Can you work these out from the model? Positions are in its coordinate system, mm. Face numbers are marked on the shaded views. Give positions to 0.01 mm unless a question says otherwise; leave off trailing zeros. Loops run counter-clockwise (first coordinate to the right, second up) from the corner with the lowest first, then second, coordinate; pieces in that order, holes last. Notation, with made-up numbers: (-7.5, 13.5) - (17.5, 13.5) arc R33 ccw to (17.5, 48.5) - close; hole circle Ø3 at (46, 32.25). An arc over 180 degrees is marked (long way). Answer as a JSON object with one key per item and string values.
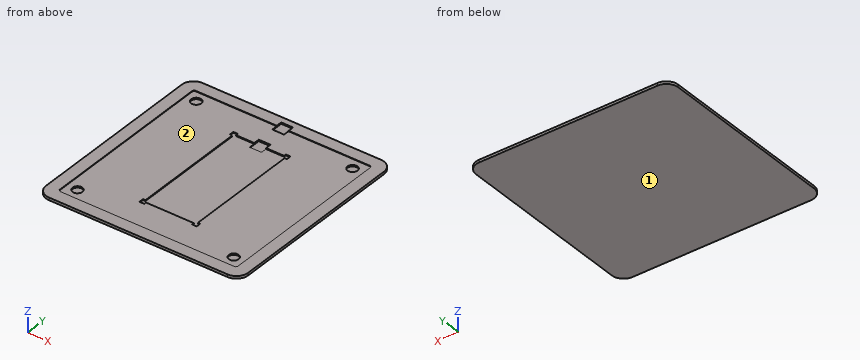
```python
from build123d import *

# Parameters (mm, degrees)
F0_W     = 10
F0_H     = 5
F1_DEPTH = 1
F2_DEPTH = 2.2
F3_DEPTH = 1.8
F4_START = 1
F4_DEPTH = 1.2
F5_START = 0.5
F5_DEPTH = 1.3
F6_R     = 4.25
F7_DEPTH = 1.2


with BuildPart() as f1:
    # F0 (on Top) → F1 (new body)
    with BuildSketch(Plane.XY):
        with BuildLine():
            Line((75.85, 85.85), (-75.85, 85.85))
            ThreePointArc((-75.85, 85.85), (-82.9210678119, 82.9210678119), (-85.85, 75.85))
            Line((-85.85, 75.85), (-85.85, -75.85))
            ThreePointArc((-85.85, -75.85), (-82.9210678119, -82.9210678119), (-75.85, -85.85))
            Line((-75.85, -85.85), (75.85, -85.85))
            ThreePointArc((75.85, -85.85), (82.9210678119, -82.9210678119), (85.85, -75.85))
            Line((85.85, -75.85), (85.85, 75.85))
            ThreePointArc((85.85, 75.85), (82.9210678119, 82.9210678119), (75.85, 85.85))
        make_face()
        with BuildLine():
            Line((5, 75.6), (73.8, 75.6))
            ThreePointArc((73.8, 75.6), (75.0727922061, 75.0727922061), (75.6, 73.8))
            Line((75.6, 73.8), (75.6, -73.8))
            ThreePointArc((75.6, -73.8), (75.0727922061, -75.0727922061), (73.8, -75.6))
            Line((73.8, -75.6), (-73.8, -75.6))
            ThreePointArc((-73.8, -75.6), (-75.0727922061, -75.0727922061), (-75.6, -73.8))
            Line((-75.6, -73.8), (-75.6, 73.8))
            ThreePointArc((-75.6, 73.8), (-75.0727922061, 75.0727922061), (-73.8, 75.6))
            Line((-73.8, 75.6), (-5, 75.6))
            Line((-5, 75.6), (-5, 80.6))
            Line((-5, 80.6), (5, 80.6))
            Line((5, 80.6), (5, 75.6))
        make_face(mode=Mode.SUBTRACT)
        with BuildLine():
            ThreePointArc((75.6, 73.8), (75.0727922061, 75.0727922061), (73.8, 75.6))
            Line((73.8, 75.6), (5, 75.6))
            Line((5, 75.6), (5, 70.6))
            Line((5, 70.6), (-5, 70.6))
            Line((-5, 70.6), (-5, 75.6))
            Line((-5, 75.6), (-73.8, 75.6))
            ThreePointArc((-73.8, 75.6), (-75.0727922061, 75.0727922061), (-75.6, 73.8))
            Line((-75.6, 73.8), (-75.6, -73.8))
            ThreePointArc((-75.6, -73.8), (-75.0727922061, -75.0727922061), (-73.8, -75.6))
            Line((-73.8, -75.6), (73.8, -75.6))
            ThreePointArc((73.8, -75.6), (75.0727922061, -75.0727922061), (75.6, -73.8))
            Line((75.6, -73.8), (75.6, 73.8))
        make_face()
        Polygon((-20.3, 52.45), (-20.3, 50.45), (-5, 50.45), (-5, 55.45), (5, 55.45), (5, 50.45), (20.3, 50.45), (20.3, 52.45), (24.3, 52.45), (24.3, 48.45), (22.3, 48.45), (22.3, -48.45), (24.3, -48.45), (24.3, -52.45), (20.3, -52.45), (20.3, -50.45), (-20.3, -50.45), (-20.3, -52.45), (-24.3, -52.45), (-24.3, -48.45), (-22.3, -48.45), (-22.3, 48.45), (-24.3, 48.45), (-24.3, 52.45), align=None, mode=Mode.SUBTRACT)
        Polygon((-5, 50.45), (-20.3, 50.45), (-20.3, 52.45), (-24.3, 52.45), (-24.3, 48.45), (-22.3, 48.45), (-22.3, -48.45), (-24.3, -48.45), (-24.3, -52.45), (-20.3, -52.45), (-20.3, -50.45), (20.3, -50.45), (20.3, -52.45), (24.3, -52.45), (24.3, -48.45), (22.3, -48.45), (22.3, 48.45), (24.3, 48.45), (24.3, 52.45), (20.3, 52.45), (20.3, 50.45), (5, 50.45), (5, 45.45), (-5, 45.45), align=None)
        with Locations((0, 78.1)):
            Rectangle(F0_W, F0_H)
        with Locations((0, 52.95)):
            Rectangle(F0_W, F0_H)
        with Locations((0, 73.1)):
            Rectangle(F0_W, F0_H)
        with Locations((0, 47.95)):
            Rectangle(F0_W, F0_H)
    extrude(amount=F1_DEPTH)

    # F0 (on Top) → F2 (join)
    with BuildSketch(Plane.XY):
        with BuildLine():
            Line((75.85, 85.85), (-75.85, 85.85))
            ThreePointArc((-75.85, 85.85), (-82.9210678119, 82.9210678119), (-85.85, 75.85))
            Line((-85.85, 75.85), (-85.85, -75.85))
            ThreePointArc((-85.85, -75.85), (-82.9210678119, -82.9210678119), (-75.85, -85.85))
            Line((-75.85, -85.85), (75.85, -85.85))
            ThreePointArc((75.85, -85.85), (82.9210678119, -82.9210678119), (85.85, -75.85))
            Line((85.85, -75.85), (85.85, 75.85))
            ThreePointArc((85.85, 75.85), (82.9210678119, 82.9210678119), (75.85, 85.85))
        make_face()
        with BuildLine():
            Line((5, 75.6), (73.8, 75.6))
            ThreePointArc((73.8, 75.6), (75.0727922061, 75.0727922061), (75.6, 73.8))
            Line((75.6, 73.8), (75.6, -73.8))
            ThreePointArc((75.6, -73.8), (75.0727922061, -75.0727922061), (73.8, -75.6))
            Line((73.8, -75.6), (-73.8, -75.6))
            ThreePointArc((-73.8, -75.6), (-75.0727922061, -75.0727922061), (-75.6, -73.8))
            Line((-75.6, -73.8), (-75.6, 73.8))
            ThreePointArc((-75.6, 73.8), (-75.0727922061, 75.0727922061), (-73.8, 75.6))
            Line((-73.8, 75.6), (-5, 75.6))
            Line((-5, 75.6), (-5, 80.6))
            Line((-5, 80.6), (5, 80.6))
            Line((5, 80.6), (5, 75.6))
        make_face(mode=Mode.SUBTRACT)
        with Locations((0, 78.1)):
            Rectangle(F0_W, F0_H)
    extrude(amount=F2_DEPTH)

    # F0 (on Top) → F3 (join)
    with BuildSketch(Plane.XY):
        with BuildLine():
            ThreePointArc((75.6, 73.8), (75.0727922061, 75.0727922061), (73.8, 75.6))
            Line((73.8, 75.6), (5, 75.6))
            Line((5, 75.6), (5, 70.6))
            Line((5, 70.6), (-5, 70.6))
            Line((-5, 70.6), (-5, 75.6))
            Line((-5, 75.6), (-73.8, 75.6))
            ThreePointArc((-73.8, 75.6), (-75.0727922061, 75.0727922061), (-75.6, 73.8))
            Line((-75.6, 73.8), (-75.6, -73.8))
            ThreePointArc((-75.6, -73.8), (-75.0727922061, -75.0727922061), (-73.8, -75.6))
            Line((-73.8, -75.6), (73.8, -75.6))
            ThreePointArc((73.8, -75.6), (75.0727922061, -75.0727922061), (75.6, -73.8))
            Line((75.6, -73.8), (75.6, 73.8))
        make_face()
        Polygon((-20.3, 52.45), (-20.3, 50.45), (-5, 50.45), (-5, 55.45), (5, 55.45), (5, 50.45), (20.3, 50.45), (20.3, 52.45), (24.3, 52.45), (24.3, 48.45), (22.3, 48.45), (22.3, -48.45), (24.3, -48.45), (24.3, -52.45), (20.3, -52.45), (20.3, -50.45), (-20.3, -50.45), (-20.3, -52.45), (-24.3, -52.45), (-24.3, -48.45), (-22.3, -48.45), (-22.3, 48.45), (-24.3, 48.45), (-24.3, 52.45), align=None, mode=Mode.SUBTRACT)
        with Locations((0, 73.1)):
            Rectangle(F0_W, F0_H)
        with Locations((0, 52.95)):
            Rectangle(F0_W, F0_H)
    extrude(amount=F3_DEPTH)

    # F0 (on Top) → F4 (cut)
    with BuildSketch(Plane.XY.offset(F4_START)):
        with Locations((0, 78.1)):
            Rectangle(F0_W, F0_H)
        with Locations((0, 73.1)):
            Rectangle(F0_W, F0_H)
    extrude(amount=F4_DEPTH, mode=Mode.SUBTRACT)

    # F0 (on Top) → F5 (cut)
    with BuildSketch(Plane.XY.offset(F5_START)):
        with Locations((0, 52.95)):
            Rectangle(F0_W, F0_H)
        with Locations((0, 47.95)):
            Rectangle(F0_W, F0_H)
    extrude(amount=F5_DEPTH, mode=Mode.SUBTRACT)

    # F6 (on face) → F7 (cut)
    with BuildSketch(Plane.XY.offset(1.8)):
        with Locations((-66.35, 66.35)):
            Circle(F6_R)
        with Locations((66.35, 66.35)):
            Circle(F6_R)
        with Locations((66.35, -66.35)):
            Circle(F6_R)
        with Locations((-66.35, -66.35)):
            Circle(F6_R)
    extrude(amount=-F7_DEPTH, mode=Mode.SUBTRACT)


solid = f1.part
```
1) I'm going to push flat-ended pins straight in: P1, Ø7, axis at x = 68, y = -65, coming from the +Z side; P2, Ø7, axis at x = -66.5, y = 66.5, coming from the +Z side. Where does each tip first touch, or does it pass through?
Check sheet entries:
{"P1": "z = 1.8", "P2": "z = 0.6"}
2) I need wall thicknesses on L1, parallel to Y at x = -66.35, z = 1.1; L2, parallel to Y at x = -17.5, z = 1.6. Which ranges of each line are inside material? Lowest first, please.
Check sheet entries:
{"L1": "-85.85 to -70.6, -62.1 to 62.1, 70.6 to 85.85", "L2": "-85.85 to -50.45, 50.45 to 85.85"}
3) Imagine slicing it at D-D on y = 29.5. Write out the boundary of the cut face in (x, z).
Check sheet entries:
{"outline": "(-85.85, 0) - (85.85, 0) - (85.85, 2.2) - (75.6, 2.2) - (75.6, 1.8) - (22.3, 1.8) - (22.3, 1) - (-22.3, 1) - (-22.3, 1.8) - (-75.6, 1.8) - (-75.6, 2.2) - (-85.85, 2.2) - close"}
4) If we mould it in two halves opening along X, with no side actions, what happens to the marked faces 1 and 2? For each: released by +X, released by -X, zero draft, split by the parting line, or undercut.
Check sheet entries:
{"face 1": "zero draft", "face 2": "undercut"}
5) Imagine slicing it at B-B on y = 66.35. Write out the boundary of the cut face in (x, z).
Check sheet entries:
{"outline": "(-85.85, 0) - (85.85, 0) - (85.85, 2.2) - (75.6, 2.2) - (75.6, 1.8) - (70.6, 1.8) - (70.6, 0.6) - (62.1, 0.6) - (62.1, 1.8) - (-62.1, 1.8) - (-62.1, 0.6) - (-70.6, 0.6) - (-70.6, 1.8) - (-75.6, 1.8) - (-75.6, 2.2) - (-85.85, 2.2) - close"}
6) Imagine slicing it at A-A on x = -38. Write out the boundary of the cut face in (y, z), and give its area (3 significant figures).
Check sheet entries:
{"outline": "(-85.85, 0) - (85.85, 0) - (85.85, 2.2) - (75.6, 2.2) - (75.6, 1.8) - (-75.6, 1.8) - (-75.6, 2.2) - (-85.85, 2.2) - close", "area": "317 mm2"}
